from build123d import *

# Parameters (mm, degrees)
F0_R     = 19.05
F1_DEPTH = 152.4
F3_D     = 228.6
F3_DEPTH = 19.051
F4_D     = 228.6


with BuildPart() as f1:
    # F0 (on Right) → F1 (new body)
    with BuildSketch(Plane.YZ):
        Circle(F0_R)
    extrude(amount=F1_DEPTH)

    # F3 (through all, one way)
    with BuildSketch(Plane.XZ):
        with Locations((0, 95.2389016747)):
            Circle(F3_D / 2)
    extrude(amount=-F3_DEPTH, mode=Mode.SUBTRACT)

    # F4 (through all)
    with Locations(Plane(origin=(0, 0, 0), x_dir=(1, 0, 0), z_dir=(0, 1, 0))):
        with Locations((0, -95.2389016747)):
            Hole(F4_D / 2)


solid = f1.part
Geometry: final body of the model. Coordinates: model frame, mm. Give positions to 0.01 mm unless a question says otherwise; leave off trailing zeros. Order: outer loops, then holes, each group sorted by start corner. A loop starts at its lowest first (then second) coordinate and runs counter-clockwise, first axis right, second up. Notation, with made-up numbers: (77.25, -24) -> (96.25, -24) arc R14 ccw to (96.25, 1) -> close; hole circle Ø3 at (-20, 54). An arc over 180 degrees is marked (long way). Write each question's results on one line, items separated by ' | '.
1) First-contact query: pin 1 Ø10 at (y, z) = (0, 9) entering from -X; pin 2 Ø10 at (x, z) = (129.5, 6) entering from -Y; pin 3 Ø10 at (y, z) = (7.5, 4.5) entering from -X. Flat tips, straight axial feed; report the tip coordinate or a pass-through.
Geometry says:
pin 1: stops at x = 68.85 | pin 2: stops at y = -19.02 | pin 3: stops at x = 62.44
2) Line query: line 1 along Y through (x, z) = (82, -14.5); line 2 along X through (y, z) = (13, -6); line 3 along X through (y, z) = (-2, -7.5). Output: solid intervals per line, ascending.
Geometry says:
line 1: y = -12.36 to 12.36 | line 2: x = 53.06 to 152.4 | line 3: x = 50.09 to 152.4
3) Cut plane D-D (x = 41). Output: boundary loops of the cut face in (y, z), and give its area (3 significant figures).
Geometry says:
outline: (-15.22, -11.45) arc R19.05 ccw to (15.22, -11.45) -> close | area: 162 mm²
4) Cut plane A-A (y = 0). Output: boundary loops of the cut face in (x, z), and give its area (3 significant figures).
Geometry says:
outline: (1.59, -19.05) -> (152.4, -19.05) -> (152.4, 19.05) -> (85.2, 19.05) arc R114.3 cw to start | area: 3,560 mm²
5) Cut plane C-C (z = -12.5). Output: boundary loops of the cut face in (x, y).
Geometry says:
outline: (38.17, -14.38) -> (152.4, -14.38) -> (152.4, 14.38) -> (38.17, 14.38) -> close
6) Cut plane B-B (x = 122). Output: boundary loops of the cut face in (y, z), and give its area (3 significant figures).
Geometry says:
outline: circle Ø38.1 at (0, 0) | area: 1,140 mm²
